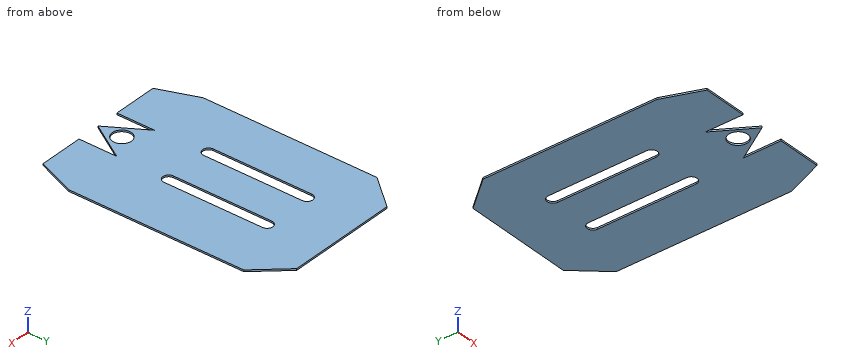
```python
from build123d import *

# Parameters (mm, degrees)
F1_DEPTH = 1
F3_DEPTH = 25
F5_DEPTH = 25
F6_DEPTH = 25
F2_R     = 5.7880952092
F7_DEPTH = 25


with BuildPart() as f1:
    # F0 (on Top) → F1 (new body)
    with BuildSketch(Plane.XY):
        Polygon((40.0670631063, 70.4256593338), (-27.2264379082, 70.4256593338), (-43.2491574436, 51.2352331091), (-43.2491574436, -54.7129847109), (-34.4047052506, -78.0962194188), (-7.5810035465, -78.0962194188), (-7.5810035465, -55.0962194188), (6.5611320772, -78.0962194188), (20.703267701, -55.0962194188), (20.703267701, -78.0962194188), (47.5269694051, -78.0962194188), (56.7508425564, -54.8600372004), (56.7508425564, 51.807079816), align=None)
    extrude(amount=F1_DEPTH)

    # F2 (on face) → F3 (cut)
    with BuildSketch(Plane.XY.offset(1)):
        with BuildLine():
            ThreePointArc((-5.9025767259, 36.2230366468), (-9.419005597, 39.7394655179), (-12.9354344681, 36.2230366468))
            Line((-12.9354344681, 36.2230366468), (-12.9354344681, -23.7769633532))
            ThreePointArc((-12.9354344681, -23.7769633532), (-9.419005597, -27.2933922242), (-5.9025767259, -23.7769633532))
            Line((-5.9025767259, -23.7769633532), (-5.9025767259, 36.2230366468))
        make_face()
    extrude(amount=-F3_DEPTH, mode=Mode.SUBTRACT)

    # F4 (on face) → F5 (cut)
    with BuildSketch(Plane.XY.offset(1)):
        with BuildLine():
            Line((16.5544010537, 35.9870965779), (16.5544010537, -24.0129034221))
            ThreePointArc((16.5544010537, -24.0129034221), (20.0195604854, -27.4780628539), (23.4847199172, -24.0129034221))
            Line((23.4847199172, -24.0129034221), (23.4847199172, 35.9870965779))
            ThreePointArc((23.4847199172, 35.9870965779), (20.0195604854, 39.4522560096), (16.5544010537, 35.9870965779))
        make_face()
    extrude(amount=-F5_DEPTH, mode=Mode.SUBTRACT)

    # F2 (on face) → F6 (cut)
    with BuildSketch(Plane.XY.offset(1)):
        with BuildLine():
            ThreePointArc((-5.9025767259, 36.2230366468), (-9.419005597, 39.7394655179), (-12.9354344681, 36.2230366468))
            Line((-12.9354344681, 36.2230366468), (-12.9354344681, -23.7769633532))
            ThreePointArc((-12.9354344681, -23.7769633532), (-9.419005597, -27.2933922242), (-5.9025767259, -23.7769633532))
            Line((-5.9025767259, -23.7769633532), (-5.9025767259, 36.2230366468))
        make_face()
    extrude(amount=-F6_DEPTH, mode=Mode.SUBTRACT)

    # F2 (on face) + F1_face1 (on face) → F7 (cut)
    with BuildSketch(Plane.XY.offset(1)):
        with BuildLine():
            ThreePointArc((-5.9025767259, 36.2230366468), (-9.419005597, 39.7394655179), (-12.9354344681, 36.2230366468))
            Line((-12.9354344681, 36.2230366468), (-12.9354344681, -23.7769633532))
            ThreePointArc((-12.9354344681, -23.7769633532), (-9.419005597, -27.2933922242), (-5.9025767259, -23.7769633532))
            Line((-5.9025767259, -23.7769633532), (-5.9025767259, 36.2230366468))
        make_face()
        with Locations((6.4631924033, -63.5865926743)):
            Circle(F2_R)
    with BuildSketch(Plane(origin=(6.8498182108, -3.4099472257, 0), x_dir=(1, 0, 0), z_dir=(0, 0, -1))):
        Polygon((33.2172448955, -73.8356065595), (49.9010243455, -55.2170270416), (49.9010243455, 51.4500899747), (40.6771511943, 74.6862721932), (13.8534494901, 74.6862721932), (13.8534494901, 51.6862721932), (-0.2886861336, 74.6862721932), (-14.4308217573, 51.6862721932), (-14.4308217573, 74.6862721932), (-41.2545234614, 74.6862721932), (-50.0989756545, 51.3030374853), (-50.0989756545, -54.6451803347), (-34.076256119, -73.8356065595), align=None)
        with BuildLine():
            Line((9.7045828429, -39.3970438035), (9.7045828429, 20.6029561965))
            ThreePointArc((9.7045828429, 20.6029561965), (13.1697422746, 24.0681156282), (16.6349017064, 20.6029561965))
            Line((16.6349017064, 20.6029561965), (16.6349017064, -39.3970438035))
            ThreePointArc((16.6349017064, -39.3970438035), (13.1697422746, -42.8622032353), (9.7045828429, -39.3970438035))
        make_face(mode=Mode.SUBTRACT)
        with BuildLine():
            Line((-12.7523949367, 20.3670161275), (-12.7523949367, -39.6329838725))
            ThreePointArc((-12.7523949367, -39.6329838725), (-16.2688238078, -43.1494127436), (-19.7852526789, -39.6329838725))
            Line((-19.7852526789, -39.6329838725), (-19.7852526789, 20.3670161275))
            ThreePointArc((-19.7852526789, 20.3670161275), (-16.2688238078, 23.8834449986), (-12.7523949367, 20.3670161275))
        make_face(mode=Mode.SUBTRACT)
    extrude(amount=-F7_DEPTH, dir=(0, 0, 1), mode=Mode.SUBTRACT)


solid = f1.part
```
Could you check a few things on this model? Use its own coordinates, in mm. Round coordinates to 2 decimals unless told otherwise and drop trailing zeros. Loops run counter-clockwise (first coordinate to the right, second up) from the corner with the lowest first, then second, coordinate; pieces in that order, holes last. Notation, with made-up numbers: M 66,52.25 L 86,52.25 A19 ccw 86,83.25 Z; hole C 46.25,-17 d10. An arc over 180 degrees is marked long. Answer as CSV lines item,"result".
1) If I drill on probe 1 along X at (y, z) = (10, 0.9); probe 2 along X at (y, z) = (-68, 0.15); probe 3 along Y at (x, z) = (-9, 0.35), over which ranges is the centre line in solid material (lowest first)?
From the geometry:
probe 1,"-43.25 to -12.94, -5.9 to 16.55, 23.48 to 56.75"
probe 2,"-38.22 to -7.58, 0.35 to 2.72, 10.21 to 12.77, 20.7 to 51.53"
probe 3,"-78.1 to -27.27, 39.71 to 70.43"
2) Imagine slicing it at D-D on y = 59. List the corners of the cut face in (x, z) for me, and give its area (3 significant figures).
From the geometry:
outline,"M -36.77,0 L 50.31,0 L 50.31,1 L -36.77,1 Z"
area,"87.1 mm^2"
3) Imagine slicing it at C-C on z = 0.2. List the corners of the cut face in (x, y) for me, and give its area (3 significant figures).
From the geometry:
outline,"M -43.25,-54.71 L -34.4,-78.1 L -7.58,-78.1 L -7.58,-55.1 L 6.56,-78.1 L 20.7,-55.1 L 20.7,-78.1 L 47.53,-78.1 L 56.75,-54.86 L 56.75,51.81 L 40.07,70.43 L -27.23,70.43 L -43.25,51.24 Z; hole M -12.94,-23.78 A3.52 ccw -5.9,-23.78 L -5.9,36.22 A3.52 ccw -12.94,36.22 Z; hole C 6.46,-63.59 d11.58; hole M 16.55,-24.01 A3.47 ccw 23.48,-24.01 L 23.48,35.99 A3.47 ccw 16.55,35.99 Z"
area,"13,000 mm^2"
4) Imagine slicing it at B-B on x = -11. List the corners of the cut face in (y, z) for me.
From the geometry:
outline,"M -78.1,0 L -26.92,0 L -26.92,1 L -78.1,1 Z; M 39.36,0 L 70.43,0 L 70.43,1 L 39.36,1 Z"
5) Imagine slicing it at A-A on y = 34.5. List the corners of the cut face in (x, z) for me, and give its area (3 significant figures).
From the geometry:
outline,"M -43.25,0 L -12.94,0 L -12.94,1 L -43.25,1 Z; M -5.9,0 L 16.55,0 L 16.55,1 L -5.9,1 Z; M 23.48,0 L 56.75,0 L 56.75,1 L 23.48,1 Z"
area,"86.0 mm^2"
